Solid Edge part; units mm, degrees
sketch "Sketch1" plane through (0, 0, 0) normal (0, -1, 0) x (1, 0, 0)
  line L0 (-12.5, -20) -> (12.5, -20)
  line L1 (12.5, -20) -> (12.5, -10)
  line L2 (12.5, 10) -> (12.5, 20)
  line L3 (12.5, 20) -> (-12.5, 20)
  line L4 (-12.5, 20) -> (-12.5, -20)
  arc A0 (12.5, -10) -> (12.5, 10) centre (12.5, 0) cw
  dimension "D1" = 12.5
  dimension "D2" = 12.5
  dimension "D3" = 12.5
extrude "Protrusion1" add sketch "Sketch1" against normal blind 210
hole "Hole_1" at (12.5, 10, 15) direction (-1, 0, 0) diameter 8.4 end up to next
hole "Hole1" at (12.5, 10, -15) direction (-1, 0, 0) diameter 8.4 end up to next
hole "Hole2" at (12.5, 105, -15) direction (-1, 0, 0) diameter 8.4 end up to next
hole "Hole3" at (12.5, 105, 15) direction (-1, 0, 0) diameter 8.4 end up to next
hole "Hole4" at (12.5, 200, 15) direction (-1, 0, 0) diameter 8.4 end up to next
hole "Hole5" at (12.5, 200, -15) direction (-1, 0, 0) diameter 8.4 end up to next
properties material "Stainless Steel, 420"
CAD build for the part. Positions are in the model's coordinates, mm. Coordinates: 2 decimals unless noted, no trailing zeros. Loops run counter-clockwise (first coordinate to the right, second up) from the corner with the lowest first, then second, coordinate; pieces in that order, holes last. Notation, with made-up numbers: (77.25, 5) - (114.25, 5) arc R33 cw to (114.25, 40) - close; hole circle Ø5 at (-25, 73.5). An arc over 180 degrees is marked (long way). Return JSON: item names as keys, results as strings.
1. Band-saw the part on D-D (x = -6.5). Give the cut face in (y, z).
Result:
{"outline": "(0, -20) - (210, -20) - (210, 20) - (0, 20) - close; hole circle Ø8.4 at (10, -15); hole circle Ø8.4 at (10, 15); hole circle Ø8.4 at (105, -15); hole circle Ø8.4 at (105, 15); hole circle Ø8.4 at (200, -15); hole circle Ø8.4 at (200, 15)"}
2. Band-saw the part on B-B (z = 15). Give the cut face in (x, y), and give its area (3 significant figures).
Result:
{"outline": "(-12.5, 0) - (12.5, 0) - (12.5, 5.8) - (-12.5, 5.8) - close; (-12.5, 14.2) - (12.5, 14.2) - (12.5, 100.8) - (-12.5, 100.8) - close; (-12.5, 109.2) - (12.5, 109.2) - (12.5, 195.8) - (-12.5, 195.8) - close; (-12.5, 204.2) - (12.5, 204.2) - (12.5, 210) - (-12.5, 210) - close", "area": "4,620 mm2"}
3. Band-saw the part on A-A (x = 9.5). Give the cut face in (y, z).
Result:
{"outline": "(0, -20) - (210, -20) - (210, -9.54) - (0, -9.54) - close; (0, 9.54) - (210, 9.54) - (210, 20) - (0, 20) - close; hole circle Ø8.4 at (10, -15); hole circle Ø8.4 at (10, 15); hole circle Ø8.4 at (105, -15); hole circle Ø8.4 at (105, 15); hole circle Ø8.4 at (200, -15); hole circle Ø8.4 at (200, 15)"}
4. Band-saw the part on C-C (y = 10). Give the cut face in (x, z), and give its area (3 significant figures).
Result:
{"outline": "(-12.5, -20) - (12.5, -20) - (12.5, -19.2) - (-12.5, -19.2) - close; (-12.5, -10.8) - (12.5, -10.8) - (12.5, -10) arc R10 cw to (12.5, 10) - (12.5, 10.8) - (-12.5, 10.8) - close; (-12.5, 19.2) - (12.5, 19.2) - (12.5, 20) - (-12.5, 20) - close", "area": "423 mm2"}
5. Mould opens along Z. For faces 1 (the flat face through (-3, 210, 0)), 2 (the cylindrical face through (0.18, 100.9, 15.91)), 3 (the flat face through (0, 104, 20)) say: released by +Z, released by -Z, zero draft, split by the parting line, or undercut.
Result:
{"face 1": "zero draft", "face 2": "undercut", "face 3": "released by +Z"}
6. Probe L1, parallel to Y at x = 3.25, z = -15; L2, parallel to Z at x = -3.25, y = 105; L3, parallel to Y at x = 6, z = 12. List the from-to ranges inside material, lowest first. Write a range as from..to.
Result:
{"L1": "y = 0..5.8, 14.2..100.8, 109.2..195.8, 204.2..210", "L2": "z = -20..-19.2, -10.8..10.8, 19.2..20", "L3": "y = 0..7.06, 12.94..102.06, 107.94..197.06, 202.94..210"}
